Read the model definition and answer for the solid it produces. Units are mm, in the model's axes. Face numbers are marked on the shaded views. Give positions to 0.01 mm unless a question says otherwise; leave off trailing zeros. Order: outer loops, then holes, each group sorted by start corner. A loop starts at its lowest first (then second) coordinate and runs counter-clockwise, first axis right, second up.
Item 1: A cutting plane is placed at C-C (y = 63). Write down the section's boundary in (x, z).
Item 2: Find the intervals of material crossed by line 1 along X through (y, z) = (58, 0); line 2 along Z through (x, y) = (-8, 74); line 3 along X through (y, z) = (71, -12), in increasing order.
Item 3: A cutting plane is placed at B-B (z = 0). Write down the section's boundary in (x, y).
Item 4: Given pin 1 Ø10 at (x, y) = (18, 24) entering from +Z; pin 2 Ø8 at (x, y) = (-18.5, 35.5) entering from +Z; pin 3 Ø2 at (y, z) = (39, -13) entering from -X, each flat-ended and moving along its own axis, determine where each tip first touches the part or whether it passes through.
Item 5: A cutting plane is placed at D-D (x = 11). Write down the section's boundary in (y, z).
Item 6: The mould has two halves that part along X. Classify the marked faces 1 and 2: +X half, -X half, draft (parallel to the pull), parting line (faces both ways), or undercut.
Item 7: A cutting plane is placed at A-A (x = 0). Write down the section's boundary in (y, z), plus the area to 3 significant figures.
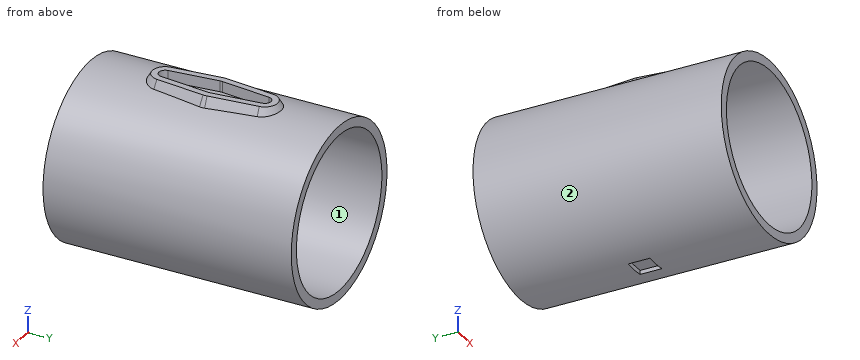
from build123d import *

# Parameters (mm, degrees)
SKETCH1_R                = 28
SKETCH1_R_2              = 25
BOSS_EXTRUDE1_DEPTH      = 80
CUT_EXTRUDE3_DEPTH       = 101.768298586
EXTRUDE_THIN2_DEPTH      = 3.5
EXTRUDE_THIN3_REACH      = 104.703
EXTRUDE_THIN3_END_RADIUS = 28
EXTRUDE_THIN3_DRAFT      = 30
SKETCH10_W               = 7
SKETCH10_H               = 7
CUT_EXTRUDE4_DEPTH       = 3


with BuildPart() as part:
    # Sketch1 → Boss-Extrude1 (new body)
    with BuildSketch(Plane(origin=(0, 0, 0), x_dir=(1, 0, 0), z_dir=(0, 1, 0))):
        with Locations(Location((0, 0, 0), (0, 0, 270))):
            Circle(SKETCH1_R)
        with Locations(Location((0, 0, 0), (0, 0, 270))):
            Circle(SKETCH1_R_2, mode=Mode.SUBTRACT)
    extrude(amount=BOSS_EXTRUDE1_DEPTH)

    # Sketch6 → Cut-Extrude3 (cut, through all)
    with BuildSketch(Plane.XY.offset(26.5)):
        with BuildLine():
            Line((-3.727642468, 40.408878505), (-1.988075983, 56.268068536))
            ThreePointArc((-1.988075983, 56.268068536), (0, 58.05), (1.988075983, 56.268068536))
            Line((1.988075983, 56.268068536), (3.727642468, 40.408878505))
            ThreePointArc((3.727642468, 40.408878505), (3.75, 40), (3.727642468, 39.591121495))
            Line((3.727642468, 39.591121495), (1.988075983, 23.731931464))
            ThreePointArc((1.988075983, 23.731931464), (0, 21.95), (-1.988075983, 23.731931464))
            Line((-1.988075983, 23.731931464), (-3.727642468, 39.591121495))
            ThreePointArc((-3.727642468, 39.591121495), (-3.75, 40), (-3.727642468, 40.408878505))
        make_face()
    extrude(amount=CUT_EXTRUDE3_DEPTH, mode=Mode.SUBTRACT)

    # Sketch7 → Extrude-Thin2 (add)
    with BuildSketch(Plane.XY.offset(26.5)):
        with BuildLine():
            Line((5.715718451, 40.62694704), (3.976151966, 56.486137072))
            ThreePointArc((3.976151966, 56.486137072), (0, 60.05), (-3.976151966, 56.486137072))
            Line((-3.976151966, 56.486137072), (-5.715718451, 40.62694704))
            ThreePointArc((-5.715718451, 40.62694704), (-5.75, 40), (-5.715718451, 39.37305296))
            Line((-5.715718451, 39.37305296), (-3.976151966, 23.513862928))
            ThreePointArc((-3.976151966, 23.513862928), (0, 19.95), (3.976151966, 23.513862928))
            Line((3.976151966, 23.513862928), (5.715718451, 39.37305296))
            ThreePointArc((5.715718451, 39.37305296), (5.75, 40), (5.715718451, 40.62694704))
        make_face()
        with BuildLine():
            Line((3.727642468, 40.408878505), (1.988075983, 56.268068536))
            ThreePointArc((1.988075983, 56.268068536), (0, 58.05), (-1.988075983, 56.268068536))
            Line((-1.988075983, 56.268068536), (-3.727642468, 40.408878505))
            ThreePointArc((-3.727642468, 40.408878505), (-3.75, 40), (-3.727642468, 39.591121495))
            Line((-3.727642468, 39.591121495), (-1.988075983, 23.731931464))
            ThreePointArc((-1.988075983, 23.731931464), (0, 21.95), (1.988075983, 23.731931464))
            Line((1.988075983, 23.731931464), (3.727642468, 39.591121495))
            ThreePointArc((3.727642468, 39.591121495), (3.75, 40), (3.727642468, 40.408878505))
        make_face(mode=Mode.SUBTRACT)
    extrude(amount=EXTRUDE_THIN2_DEPTH)

    # Extrude-Thin3: up to this cylinder (the profile starts outside it)
    extrude_thin3_end = Plane(origin=(0, 48.56287, 0), z_dir=(0, -1, 0)) * Cylinder(EXTRUDE_THIN3_END_RADIUS, 266.406, mode=Mode.PRIVATE)



with BuildPart() as extrude_thin3_long_prism_1:
    # Sketch9 → Extrude-Thin3 (the long prism of profile 1, to be tilted and cut off)
    with BuildSketch(Plane.XY.offset(30)):
        with BuildLine():
            Line((-4.075555765, 56.497040498), (-5.81512225, 40.637850467))
            ThreePointArc((-5.81512225, 40.637850467), (-5.85, 40), (-5.81512225, 39.362149533))
            Line((-5.81512225, 39.362149533), (-4.075555765, 23.502959502))
            ThreePointArc((-4.075555765, 23.502959502), (0, 19.85), (4.075555765, 23.502959502))
            Line((4.075555765, 23.502959502), (5.81512225, 39.362149533))
            ThreePointArc((5.81512225, 39.362149533), (5.85, 40), (5.81512225, 40.637850467))
            Line((5.81512225, 40.637850467), (4.075555765, 56.497040498))
            ThreePointArc((4.075555765, 56.497040498), (0, 60.15), (-4.075555765, 56.497040498))
        make_face()
        with BuildLine():
            Line((-3.976151966, 56.486137072), (-5.715718451, 40.62694704))
            ThreePointArc((-5.715718451, 40.62694704), (-5.75, 40), (-5.715718451, 39.37305296))
            Line((-5.715718451, 39.37305296), (-3.976151966, 23.513862928))
            ThreePointArc((-3.976151966, 23.513862928), (0, 19.95), (3.976151966, 23.513862928))
            Line((3.976151966, 23.513862928), (5.715718451, 39.37305296))
            ThreePointArc((5.715718451, 39.37305296), (5.75, 40), (5.715718451, 40.62694704))
            Line((5.715718451, 40.62694704), (3.976151966, 56.486137072))
            ThreePointArc((3.976151966, 56.486137072), (0, 60.05), (-3.976151966, 56.486137072))
        make_face(mode=Mode.SUBTRACT)
    extrude(amount=-EXTRUDE_THIN3_REACH)
    extrude_thin3_tool1_sides = [extrude_thin3_long_prism_1.faces().sort_by_distance(p)[0] for p in [
        (4.945339007, 48.567445483, -22.3515),
        (0, 60.15, -22.3515),
        (-4.945339007, 48.567445483, -22.3515),
        (-5.85, 40, -22.3515),
        (-4.945339007, 31.432554517, -22.3515),
        (0, 19.85, -22.3515),
        (4.945339007, 31.432554517, -22.3515),
        (5.85, 40, -22.3515),
        (4.845935208, 48.556542056, -22.3515),
        (5.75, 40, -22.3515),
        (4.845935208, 31.443457944, -22.3515),
        (0, 19.95, -22.3515),
        (-4.845935208, 31.443457944, -22.3515),
        (-5.75, 40, -22.3515),
        (-4.845935208, 48.556542056, -22.3515),
        (0, 60.05, -22.3515),
    ]]
    draft(extrude_thin3_tool1_sides, Plane.XY.offset(30), EXTRUDE_THIN3_DRAFT)  # the draft: side faces tilted about the start plane


with BuildPart() as part_1:
    add(part.part)
    extrude_thin3_tool1 = extrude_thin3_long_prism_1.part - extrude_thin3_end
    add(extrude_thin3_tool1.solids().sort_by_distance((4.903625, 48.56287, 30))[0])

    # Sketch10 → Cut-Extrude4 (cut)
    with BuildSketch(Plane.XY.offset(-26.5)):
        with Locations((0, 40)):
            Rectangle(SKETCH10_W, SKETCH10_H)
    extrude(amount=-CUT_EXTRUDE4_DEPTH, mode=Mode.SUBTRACT)


solid = part_1.part
Response values:
1. outline: circle Ø56 at (0, 0); hole circle Ø50 at (0, 0)
2. line 1: x = -28 to -25, 25 to 28
2. line 2: z = -26.83 to -23.69, 23.69 to 26.83
2. line 3: x = -25.3 to -21.93, 21.93 to 25.3
3. outline: (-28, 0) - (-25, 0) - (-25, 80) - (-28, 80) - close; (25, 0) - (28, 0) - (28, 80) - (25, 80) - close
4. pin 1: stops at z = 24.8
4. pin 2: stops at z = 23.95
4. pin 3: stops at x = -25.3
5. outline: (0, -25.75) - (80, -25.75) - (80, -22.45) - (0, -22.45) - close; (0, 22.45) - (80, 22.45) - (80, 25.75) - (0, 25.75) - close
6. face 1: undercut
6. face 2: parting line
7. outline: (0, -28) - (36.5, -28) - (36.5, -26.5) - (43.5, -26.5) - (43.5, -28) - (80, -28) - (80, -25) - (0, -25) - close; (0, 25) - (80, 25) - (80, 28) - (61.3, 28) - (60.15, 30) - (58.05, 30) - (58.05, 26.5) - (21.95, 26.5) - (21.95, 30) - (19.85, 30) - (18.7, 28) - (0, 28) - close
7. area: 426 mm2
